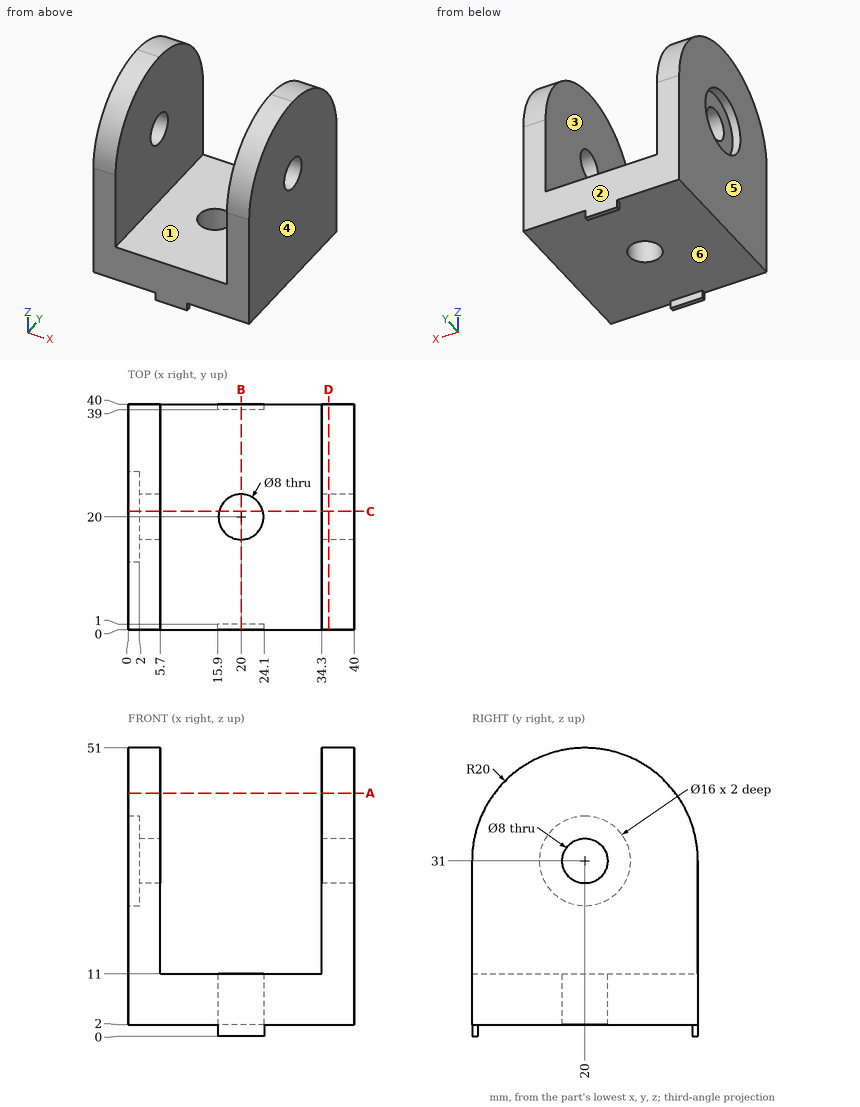
Input: dimensioned drawing with shaded views. Units: mm. Origin: part minimum x, y, z. A direction names the side the tool comes from. Give positions to 0.01 mm unless a question says otherwise; leave off trailing zeros. Loops run counter-clockwise (first coordinate to the right, second up) from the corner with the lowest first, then second, coordinate; pieces in that order, holes last. Notation, with made-up numbers: (83.25, -32.5) -> (91.25, -32.5) arc R7 cw to (91.25, -24.5) -> close; hole circle Ø4 at (68.25, -25.75). An arc over 180 degrees is marked (long way). Return JSON: item names as keys, results as strings.
Item 1: Section C-C, the plane y = 21. Output: boundary loops of the cut face in (x, z).
Filled in:
{"outline": "(0, 2) -> (16.13, 2) -> (16.13, 11) -> (5.7, 11) -> (5.7, 27.13) -> (2, 27.13) -> (2, 23.06) -> (0, 23.06) -> close; (0, 38.94) -> (2, 38.94) -> (2, 34.87) -> (5.7, 34.87) -> (5.7, 50.97) -> (0, 50.97) -> close; (23.87, 2) -> (40, 2) -> (40, 27.13) -> (34.3, 27.13) -> (34.3, 11) -> (23.87, 11) -> close; (34.3, 34.87) -> (40, 34.87) -> (40, 50.97) -> (34.3, 50.97) -> close"}
Item 2: Section D-D, the plane x = 35.5. Output: boundary loops of the cut face in (y, z).
Filled in:
{"outline": "(0, 2) -> (40, 2) -> (40, 31) arc R20 ccw to (0, 31) -> close; hole circle Ø8 at (20, 31)"}
Item 3: Pin query (flat end, axial travel): P1, Ø13, axis at y = 23, z = 31, coming from the -X side; P2, Ø13, axis at y = 20, z = 31, coming from the -X side; P3, Ø6, axis at x = 23, y = 16, coming from the -Z side; P4, Ø0.8, axis at y = 39.5, z = 1, coming from the +X side. Return the tip coordinate at first contact, or that it passes through.
Filled in:
{"P1": "x = 0", "P2": "x = 2", "P3": "z = 2", "P4": "x = 24.1"}
Item 4: Access query for the marked faces 1 and 2. Directions: +Z, -Z, +X, -X, +Y, -Y. A direction counts if a zero-diameter tool reaches every point of the face in a straight line with its end or side. Return the directions, or none.
Filled in:
{"face 1": "+Z, +Y, -Y", "face 2": "+Z, -Z, +X, -X, +Y"}
Item 5: Section A-A, the plane z = 43. Output: boundary loops of the cut face in (x, y), plus the area to 3 significant figures.
Filled in:
{"outline": "(0, 4) -> (5.7, 4) -> (5.7, 36) -> (0, 36) -> close; (34.3, 4) -> (40, 4) -> (40, 36) -> (34.3, 36) -> close", "area": "365 mm^2"}
Item 6: Line query: line 1 (Y direction, x = 2.9, z = 31); line 2 (X direction, y = 30, z = 47.5); line 3 (Y direction, x = 0.55, z = 31). Output: solid intervals per line, ascending.
Filled in:
{"line 1": "0 to 16, 24 to 40", "line 2": "0 to 5.7, 34.3 to 40", "line 3": "0 to 12, 28 to 40"}
Item 7: Section B-B, the plane x = 20. Output: boundary loops of the cut face in (y, z).
Filled in:
{"outline": "(0, 0) -> (1, 0) -> (1, 2) -> (16, 2) -> (16, 11) -> (0, 11) -> close; (24, 2) -> (39, 2) -> (39, 0) -> (40, 0) -> (40, 11) -> (24, 11) -> close"}
Item 8: Mould query, pull axis X, two halves, no side actions, for the marked faces 3, 4, 5 and 6. Classes: released by +X, released by -X, zero draft, split by the parting line, or undercut.
Filled in:
{"face 3": "undercut", "face 4": "released by +X", "face 5": "released by -X", "face 6": "zero draft"}
